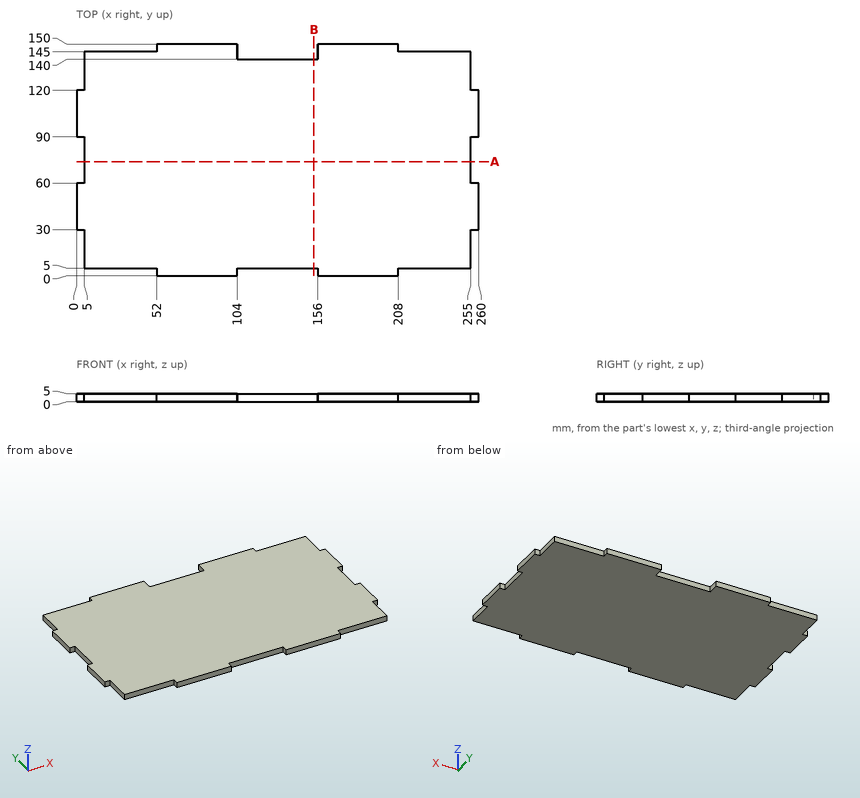
The drawing under review shows one solid part. Ordinate dimensions are in mm from its lowest x, y, z. Round coordinates to 2 decimals unless told otherwise and drop trailing zeros. Loops run counter-clockwise (first coordinate to the right, second up) from the corner with the lowest first, then second, coordinate; pieces in that order, holes last.
Item 1: Take a section at B-B (x = 153.5). Write out the cut boundary in (y, z), then the cut area to 3 significant figures.
Determined:
outline: (5, 0) - (140, 0) - (140, 5) - (5, 5) - close
area: 675 mm2
Item 2: For line 1 (X direction, y = 139, z = 1.1); line 2 (Y direction, x = 224.5, z = 0.3); line 3 (Y direction, x = 120, z = 4.65), list the stretches that pass through material, from the lowest coordinate up.
Determined:
line 1: x = 5 to 255
line 2: y = 5 to 145
line 3: y = 5 to 140
Item 3: Clearance check with flat-ended pins moving along their axes: pin 1 Ø1.5 at (x, z) = (220, 2) entering from +Y; pin 2 Ø1.5 at (y, z) = (3.5, 2.5) entering from -X; pin 3 Ø2.5 at (x, z) = (233.5, 2) entering from -Y; pin 4 Ø2 at (x, z) = (57.5, 2.5) entering from -Y. State where each tip first meets the part, or that it passes through.
Determined:
pin 1: stops at y = 145
pin 2: stops at x = 52
pin 3: stops at y = 5
pin 4: stops at y = 0
Item 4: Take a section at A-A (y = 74). Write out the cut boundary in (x, z).
Determined:
outline: (5, 0) - (255, 0) - (255, 5) - (5, 5) - close
